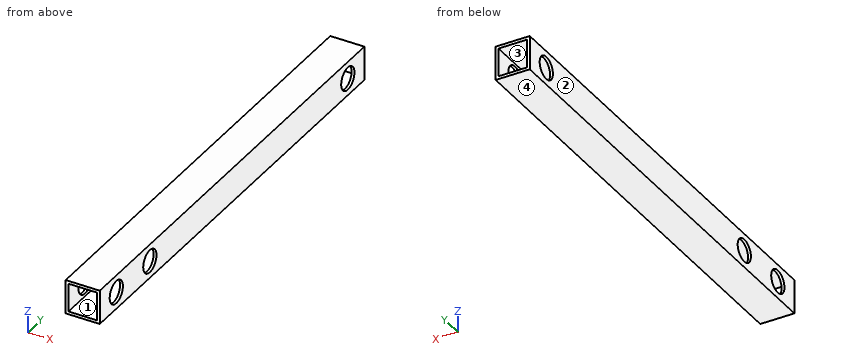
Autodesk Inventor part; units mm, degrees
ref_plane "YZ Plane" through (0, 0, 0) normal (1, 0, 0) x (0, 1, 0)
ref_plane "XZ Plane" through (0, 0, 0) normal (0, 1, 0) x (-1, 0, 0)
ref_plane "XY Plane" through (0, 0, 0) normal (0, 0, 1) x (1, 0, 0)
sketch "Boceto1" plane through (0, 0, 0) normal (0, 1, 0) x (-1, 0, 0)
  line L0 (0, 0) -> (-10, 0)
  line L1 (-10, 0) -> (-10, -10)
  line L2 (-10, -10) -> (0, -10)
  line L3 (0, -10) -> (0, 0)
  line L4 (1, 1) -> (-11, 1)
  line L5 (-11, 1) -> (-11, -11)
  line L6 (-11, -11) -> (1, -11)
  line L7 (1, -11) -> (1, 1)
  dimension "d0" = 10
  dimension "d2" = 12
  dimension "d4" = 1
  dimension "d5" = 1
extrude "Extrusión1" add sketch "Boceto1" along normal blind 160
sketch "Boceto2" plane through (-1, 0, -11) normal (-1, 0, 0) x (0, 0, 1)
  circle A0 centre (6, 10) radius 4
  circle A1 centre (6, 30.28) radius 4
  line L0 (0, 0) -> (12, 0)
  line L1 (0, 0) -> (0, 160)
  circle A2 centre (6, 150) radius 4
  line L2 (0, 160) -> (12, 160)
  dimension "d8" = 8
  dimension "d9" = 8
  dimension "d11" = 20.28
  dimension "d14" = 10
  dimension "d15" = 6
  dimension "d16" = 6
  dimension "d17" = 8
  dimension "d18" = 6
  dimension "d19" = 10
extrude "Extrusión2" cut sketch "Boceto2" against normal blind 20
properties part number "brazo"
Work out the finished part from the listing and answer in its coordinate system (mm). Face numbers are marked on the shaded views. Give positions to 0.01 mm unless a question says otherwise; leave off trailing zeros. Write each loop counter-clockwise with the first axis right and the second up, starting at its lowest first coordinate (ties: lowest second). Pieces come first, ordered by that corner, then holes.
(1) The mould has two halves that part along Z. Classify the marked faces 1, 2, 3 and 4: pulls with the +Z half, pulls with the -Z half, needs draft (parallel to the pull), parting line crosses it, or undercut.
Final values:
face 1: undercut
face 2: needs draft
face 3: undercut
face 4: pulls with the -Z half
(2) The part is cut by section C-C on y = 65. Write down the section's boundary in (x, z), plus the area to 3 significant figures.
Final values:
outline: (-1, -11) - (11, -11) - (11, 1) - (-1, 1) - close; hole (0, -10) - (10, -10) - (10, 0) - (0, 0) - close
area: 44.0 mm2
(3) The part is cut by section B-B on z = -5. Count the separate pieces of the cut face and the enclosed holes in it, plus the area to 3 significant figures.
Final values:
separate pieces: 8
enclosed holes: 0
area: 272 mm2
(4) The part is cut by section A-A on x = 6. Write down the section's boundary in (y, z).
Final values:
outline: (0, -11) - (160, -11) - (160, -10) - (0, -10) - close; (0, 0) - (160, 0) - (160, 1) - (0, 1) - close
(5) The part is cut by section D-D on y = 30.28. Write down the section's boundary in (x, z).
Final values:
outline: (-1, -11) - (11, -11) - (11, -9) - (10, -9) - (10, -10) - (0, -10) - (0, -9) - (-1, -9) - close; (-1, -1) - (0, -1) - (0, 0) - (10, 0) - (10, -1) - (11, -1) - (11, 1) - (-1, 1) - close
(6) Straight lines are drawn through the part: line 1 (Y direction, x = -0.6, z = -5); line 2 (Z direction, x = 6, y = 62); line 3 (X direction, y = 18.5, z = -4.5). For each, find the intervals that lie inside material, in ascending order.
Final values:
line 1: y = 0 to 6, 14 to 26.28, 34.28 to 146, 154 to 160
line 2: z = -11 to -10, 0 to 1
line 3: x = -1 to 0, 10 to 11
(7) Flat-ended cylindrical pins translate along their axes: pin 1 Ø7 at (y, z) = (10, -5) entering from +X; pin 2 Ø6 at (x, z) = (7, -1) entering from -Y. Find the tip coordinate at first contact, or state that the pin passes through.
Final values:
pin 1: passes through
pin 2: stops at y = 0
